Autodesk Inventor part; units mm, degrees
ref_plane "YZ Plane" through (0, 0, 0) normal (1, 0, 0) x (0, 1, 0)
ref_plane "XZ Plane" through (0, 0, 0) normal (0, 1, 0) x (-1, 0, 0)
ref_plane "XY Plane" through (0, 0, 0) normal (0, 0, 1) x (1, 0, 0)
sketch "Esboço1" plane through (0, 0, 0) normal (0, 0, 1) x (1, 0, 0)
  line L0 (-220.4936, -60.1777) -> (-220.4936, -0.1777)
  line L1 (219.5064, -0.1777) -> (219.5064, -60.1777)
  line L2 (224.5064, -60.1777) -> (224.5064, 4.8223)
  line L3 (-225.4936, 4.8223) -> (-225.4936, -60.1777)
  line L4 (-225.4936, 4.8223) -> (-225.4936, 74.8223)
  line L5 (-225.4936, 74.8223) -> (224.5064, 74.8223)
  line L6 (224.5064, 74.8223) -> (224.5064, 4.8223)
  line L7 (219.5064, -60.1777) -> (219.5064, 4.8223)
  line L8 (219.5064, 4.8223) -> (219.5064, 69.8223)
  line L9 (219.5064, 69.8223) -> (-220.4936, 69.8223)
  line L10 (-220.4936, 69.8223) -> (-220.4936, 4.8223)
  line L11 (-220.4936, 4.8223) -> (-220.4936, -60.1777)
  line L12 (-220.4936, -60.1777) -> (-225.4936, -60.1777)
  line L13 (224.5064, -60.1777) -> (219.5064, -60.1777)
  point P0 (0, 0)
  dimension "d0" = 60
  dimension "d1" = 440
  dimension "d2" = 70
  dimension "d3" = 5
extrude "Extrusão1" add sketch "Esboço1" along normal blind 2800
sketch "Esboço2" plane through (224.5064, -60.1777, 0) normal (1, 0, 0) x (0, 0, -1)
  line L0 (0, 0) -> (-2800, 0)
  line L1 (0, 0) -> (-2800, 0)
  line L2 (-2800, 0) -> (-2800, 40)
  line L3 (-2800, 40) -> (0, 40)
  line L4 (0, 40) -> (0, 0)
  circle A0 centre (-200, 20) radius 5
  circle A1 centre (-1000, 20) radius 5
  circle A2 centre (-1800, 20) radius 5
  circle A3 centre (-2600, 20) radius 5
  point P0 (0, 60.1777)
  dimension "d6" = 2800
  dimension "d7" = 40
  dimension "d8" = 10
  dimension "d9" = 10
  dimension "d10" = 10
  dimension "d11" = 10
  dimension "d12" = 20
  dimension "d13" = 20
  dimension "d14" = 20
  dimension "d15" = 20
  dimension "d16" = 800
  dimension "d17" = 800
  dimension "d18" = 800
  dimension "d19" = 200
extrude "Extrusão2" cut sketch "Esboço2" against normal through all contours A0 | A1 | A2 | A3
properties part number "Teste Placa" material "Policarbonato, transparente"
Verification items for the finished model (mm, model axes). A direction names the side the tool comes from. Give positions to 0.01 mm unless a question says otherwise; leave off trailing zeros. Loops run counter-clockwise (first coordinate to the right, second up) from the corner with the lowest first, then second, coordinate; pieces in that order, holes last.
1. Release check for a two-part mould opening along X. For faces 3 (the flat face through (-225.494, 8, 1380)), 4 (the flat face through (-220.494, 4, 1380)), 5 (the flat face through (-2, 73, 0)) record: +X half, -X half, draft (parallel to the pull), parting line (faces both ways), or undercut.
Derived:
face 3: -X half
face 4: undercut
face 5: draft
2. Tool access check on faces 1 (the flat face through (-4, 74.822, 1380)), 2 (the flat face through (3, 69.822, 1380)). Record the directions out of +Z, -Z, +X, -X, +Y, -Y that give a thin tool (end or side, any length) a straight path to the whole face; none if there is none.
Derived:
face 1: +Z, -Z, +X, -X, +Y
face 2: +Z, -Z, -Y
3. Cross-section at A-A on y = 25. Record the cut outline in (x, z).
Derived:
outline: (-225.49, 0) - (-220.49, 0) - (-220.49, 2800) - (-225.49, 2800) - close; (219.51, 0) - (224.51, 0) - (224.51, 2800) - (219.51, 2800) - close
4. Material ranges on probe 1 along X at (y, z) = (-16, 1291); probe 2 along Y at (x, z) = (-221.6, 1800); probe 3 along Y at (x, z) = (-35.5, 269.5), recorded low to high.
Derived:
probe 1: x = -225.49 to -220.49, 219.51 to 224.51
probe 2: y = -60.18 to -45.18, -35.18 to 74.82
probe 3: y = 69.82 to 74.82
5. Go/stop test with flat-tipped pins: P1, Ø8, axis at y = -40.18, z = 2600, coming from the -X side; P2, Ø3, axis at x = -67.5, z = 1545.5, coming from the -Y side. Record where each tip stops, or that it passes through.
Derived:
P1: passes through
P2: stops at y = 69.82
6. Cross-section at C-C on x = -149. Record the cut outline in (y, z).
Derived:
outline: (69.82, 0) - (74.82, 0) - (74.82, 2800) - (69.82, 2800) - close
7. Cross-section at B-B on z = 1978. Record the cut outline in (x, y), and give its area (3 significant figures).
Derived:
outline: (-225.49, -60.18) - (-220.49, -60.18) - (-220.49, 69.82) - (219.51, 69.82) - (219.51, -60.18) - (224.51, -60.18) - (224.51, 74.82) - (-225.49, 74.82) - close
area: 3,550 mm2
